Autodesk Inventor part; units mm, degrees
ref_plane "YZ Plane" through (0, 0, 0) normal (1, 0, 0) x (0, 1, 0)
ref_plane "XZ Plane" through (0, 0, 0) normal (0, 1, 0) x (-1, 0, 0)
ref_plane "XY Plane" through (0, 0, 0) normal (0, 0, 1) x (1, 0, 0)
sketch "Sketch1" plane through (0, 0, 0) normal (0, 0, 1) x (1, 0, 0)
  line L0 (-18.5, -12.375) -> (18.5, -12.375)
  line L1 (18.5, -12.375) -> (18.5, 12.375)
  line L2 (18.5, 12.375) -> (-18.5, 12.375)
  line L3 (-18.5, 12.375) -> (-18.5, -12.375)
  line L4 (-18.5, -12.375) -> (18.5, 12.375) construction
  line L5 (18.5, -12.375) -> (-18.5, 12.375) construction
  point P0 (0, 0)
  dimension "d0" = 37
  dimension "d1" = 24.75
extrude "Extrusion1" add sketch "Sketch1" along normal blind 7
sketch "Sketch2" plane through (18.5, -12.375, 0) normal (1, 0, 0) x (0, 0, -1)
  circle A0 centre (-3.5, 3.425) radius 1.5
  line L0 (-7, 0) -> (-7, 24.75)
  line L1 (0, 0) -> (-7, 0)
  point P0 (0, 12.375)
  point P1 (-3.5, 0)
  dimension "d4" = 3
  dimension "d5" = 3.5
  dimension "d6" = 3.425
hole "Hole1" at (18.5, -8.95, 3.5) direction (-1, 0, 0) diameter 3 depth 5 tip angle 118
mirror "Mirror1" about plane through (0, 0, 0) normal (0, 1, 0) of "Hole1"
mirror "Mirror2" about plane through (0, 0, 0) normal (1, 0, 0) of "Hole1", "Mirror1"
sketch "Sketch3" plane through (0, 0, 7) normal (0, 0, 1) x (1, 0, 0)
  circle A0 centre (6.8, 0) radius 1.5
  line L0 (18.5, 12.375) -> (-18.5, 12.375)
  line L1 (18.5, -12.375) -> (18.5, 12.375)
  point P0 (0, 0)
  dimension "d14" = 3
  dimension "d15" = 12.375
  dimension "d16" = 11.7
hole "Hole2" at (6.8, 0, 7) direction (0, 0, -1) diameter 3 end through all
mirror "Mirror3" about plane through (0, 0, 0) normal (1, 0, 0) of "Hole2"
sketch "Sketch4" plane through (-18.5, -12.375, 0) normal (0, -1, 0) x (1, 0, 0)
  circle A0 centre (18.9, 3.5) radius 1.5
  line L0 (0, 7) -> (37, 7)
  line L1 (0, 0) -> (0, 7)
  point P0 (18.5, 0)
  dimension "d24" = 3
  dimension "d25" = 3.5
  dimension "d26" = 18.9
hole "Hole3" at (0.4, -12.375, 3.5) direction (0, 1, 0) diameter 3 depth 5 tip angle 118
properties part number "Mold_BackWall"
Build history of the part. All positions in model axes, mm. A direction names the side the tool comes from. Give positions to 0.01 mm unless a question says otherwise; leave off trailing zeros. Loops run counter-clockwise (first coordinate to the right, second up) from the corner with the lowest first, then second, coordinate; pieces in that order, holes last.
Item 1: Flat gauge pins, fed straight in: pin 1 (3.5 mm diameter, centred on y = -8.95, z = 3.5, fed in from -X); pin 2 (2.5 mm diameter, centred on y = 8.95, z = 3.5, fed in from +X); pin 3 (2.5 mm diameter, centred on x = -6.8, y = 0, fed in from -Z). Where does each tip first touch, or does it go through?
Answers follow:
pin 1: stops at x = -18.5
pin 2: stops at x = 13.35
pin 3: passes through
Item 2: Pull direction Y, two halves, no side cores. Call faces 1 (the face through (0, 12.375, 3)), 2 (the face through (-12.755, 8.692, 3.534)), 3 (the face through (-0.3, -12.375, 5)), 4 (the face through (-18.5, 0, 3)): released by +Y, released by -Y, zero draft, split by the parting line, or undercut.
Answers follow:
face 1: released by +Y
face 2: undercut
face 3: released by -Y
face 4: zero draft
Item 3: Drill centre lines: line 1 (Y direction, x = 17.2, z = 3.5) (3 decimals); line 2 (X direction, y = 0, z = 4.5); line 3 (Y direction, x = -6.8, z = 3) (3 decimals). Where is each one in solid material? Low to high.
Answers follow:
line 1: y = -12.375 to -10.45, -7.45 to 7.45, 10.45 to 12.375
line 2: x = -18.5 to -8.3, -5.3 to 5.3, 8.3 to 18.5
line 3: y = -12.375 to -1.5, 1.5 to 12.375
Item 4: Which spindle directions (+Z, -Z, +X, -X, +Y, -Y) get a long thin tool onto all of the face, cutting with end or side? Do faces 5 (the face through (-15.965, -9.525, 2.114)), 6 (the face through (-0.05, -9.84, 2.07)), 7 (the face through (0, 0, 7)), 8 (the face through (15.96, -7.62, 2.81)). Say none if no direction does.
Answers follow:
face 5: -X
face 6: -Y
face 7: +Z, +X, -X, +Y, -Y
face 8: +X
Item 5: Slice it at D-D, the plane x = 7.5. List the corners of the cut face in (y, z) (3 decimals), and give its area (3 significant figures).
Answers follow:
outline: (-12.375, 0) - (-1.327, 0) - (-1.327, 7) - (-12.375, 7) - close; (1.327, 0) - (12.375, 0) - (12.375, 7) - (1.327, 7) - close
area: 155 mm2
Item 6: Slice it at B-B, the plane x = 15. List the corners of the cut face in (y, z) (3 decimals).
Answers follow:
outline: (-12.375, 0) - (12.375, 0) - (12.375, 7) - (-12.375, 7) - close; hole circle Ø3 at (-8.95, 3.5); hole circle Ø3 at (8.95, 3.5)
Item 7: Slice it at A-A, the plane x = -6.8. List the corners of the cut face in (y, z) (3 decimals).
Answers follow:
outline: (-12.375, 0) - (-1.5, 0) - (-1.5, 7) - (-12.375, 7) - close; (1.5, 0) - (12.375, 0) - (12.375, 7) - (1.5, 7) - close
Item 8: Slice it at C-C, the plane z = 6. List the corners of the cut face in (x, y) (3 decimals), and give its area (3 significant figures).
Answers follow:
outline: (-18.5, -12.375) - (18.5, -12.375) - (18.5, 12.375) - (-18.5, 12.375) - close; hole circle Ø3 at (-6.8, 0); hole circle Ø3 at (6.8, 0)
area: 902 mm2
